from build123d import *

# Parameters (mm, degrees)
SKETCH1_W               = 1.5
SKETCH1_H               = 31
SKETCH1_W_2             = 2.5
SKETCH1_H_2             = 16
BOSS_EXTRUDE1_DEPTH     = 20
SKETCH2_W               = 70
SKETCH2_H               = 36
BOSS_EXTRUDE2_DEPTH     = 3
CUT_EXTRUDE1_DEPTH      = 82.215762017
CUT_EXTRUDE1_DEPTH_BACK = 82.215762017


with BuildPart() as part:
    # Sketch1 → Boss-Extrude1 (new body)
    with BuildSketch(Plane(origin=(0, 0, 0), x_dir=(1, 0, 0), z_dir=(0, 1, 0))):
        Polygon((70, 36), (0, 36), (0, 33.5), (68.5, 33.5), (70, 33.5), align=None)
        with Locations((69.25, 18)):
            Rectangle(SKETCH1_W, SKETCH1_H)
        Polygon((70, 0), (70, 2.5), (68.5, 2.5), (0, 2.5), (0, 0), align=None)
        with Locations((1.25, 18)):
            Rectangle(SKETCH1_W_2, SKETCH1_H_2)
    extrude(amount=BOSS_EXTRUDE1_DEPTH)

    # Sketch2 → Boss-Extrude2 (add)
    with BuildSketch(Plane.XZ):
        with Locations((35, -18)):
            Rectangle(SKETCH2_W, SKETCH2_H)
    extrude(amount=BOSS_EXTRUDE2_DEPTH)

    # Sketch3 → Cut-Extrude1 (cut, two sides: drawn at the far end of the back side and taken through both)
    with BuildSketch(Plane.XY.offset(-CUT_EXTRUDE1_DEPTH_BACK)):
        with BuildLine():
            Line((15, 3), (20, 3))
            ThreePointArc((20, 3), (21.5, 1.5), (20, 0))
            Line((20, 0), (15, 0))
            ThreePointArc((15, 0), (13.5, 1.5), (15, 3))
        make_face()
        with BuildLine():
            Line((55, 3), (50, 3))
            ThreePointArc((50, 3), (48.5, 1.5), (50, 0))
            Line((50, 0), (55, 0))
            ThreePointArc((55, 0), (56.5, 1.5), (55, 3))
        make_face()
    extrude(amount=CUT_EXTRUDE1_DEPTH + CUT_EXTRUDE1_DEPTH_BACK, mode=Mode.SUBTRACT)


solid = part.part
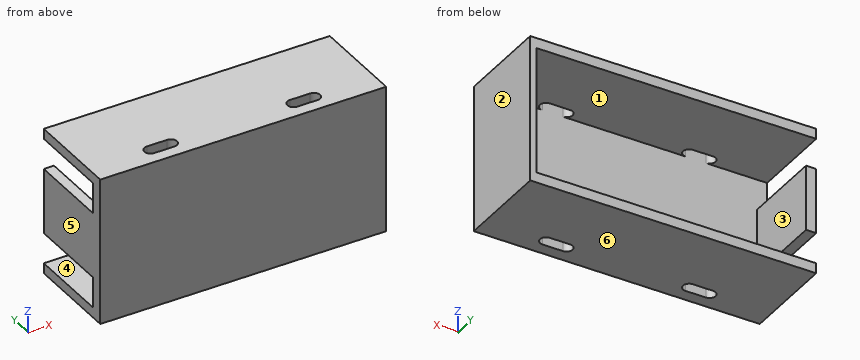
Here's how the part is built. I have some questions about the finished solid (model axes, mm). Face numbers are marked on the shaded views. A direction names the side the tool comes from. Coordinates: 2 decimals unless noted, no trailing zeros. Loops run counter-clockwise (first coordinate to the right, second up) from the corner with the lowest first, then second, coordinate; pieces in that order, holes last. Notation, with made-up numbers: (9, 87.5) -> (57, 87.5) arc R35 cw to (57, 121.5) -> close; hole circle Ø7 at (38, -27). An arc over 180 degrees is marked (long way). Use one line per item in the form item = value. Start each with the question number.
(1) If we section it at D-D (z = -4): Please give me the cut outline in (x, y).
(2) If we section it at C-C (x = 7): Please give me the cut outline in (y, z).
(3) We'd pull the mould along Z, two halves only. Please class the marked faces 4, 5 and 6: pulls with the +Z half, pulls with the -Z half, needs draft (parallel to the pull), parting line crosses it, or undercut.
(4) On a 3-axis mill with a long thin cutter (end or side, diameter ignored), from which of +Z, -Z, +X, -X, +Y, -Y can I reach the whole of each face in a straight line? I mean the marked faces 1, 2 and 3. Say none if no direction works.
(5) If we section it at A-A (y = 1.5): Please give me the cut outline in (x, z), then the cut area to 4 significant figures.
(6) If we section it at B-B (y = 18.25): Please give me the cut outline in (x, z), then the cut area to 4 significant figures.
(7) Please list where these lines run through material, in increasing order: line 1 along Z through (x, y) = (62, 14); line 2 along X through (y, z) = (1.5, -22.5); line 3 along Y through (x, z) = (49, -15).
(8) Will these pins go through, and if not, where does the flat tip stop? pin 1 (8 mm diameter, centred on x = 35.5, z = -13, fed in from +Y); pin 2 (3 mm diameter, centred on x = 1, y = 12.5, fed in from +Z); pin 3 (1 mm diameter, centred on y = 7, z = -27.5, fed in from -X).
Verdict:
q1.outline = (0, -3) -> (70, -3) -> (70, 20) -> (68.5, 20) -> (68.5, 0) -> (0, 0) -> close
q2.outline = (-3, -36) -> (20, -36) -> (20, -33.5) -> (0, -33.5) -> (0, -2.5) -> (20, -2.5) -> (20, 0) -> (-3, 0) -> close
q3.face_4 = undercut
q3.face_5 = needs draft
q3.face_6 = pulls with the -Z half
q4.face_1 = -X, +Y
q4.face_2 = +Z, -Z, +X, +Y, -Y
q4.face_3 = +Y
q5.outline = (0, -36) -> (13.5, -36) -> (13.5, -33.5) -> (0, -33.5) -> close; (0, -26) -> (2.5, -26) -> (2.5, -10) -> (0, -10) -> close; (0, -2.5) -> (13.5, -2.5) -> (13.5, 0) -> (0, 0) -> close; (21.5, -36) -> (48.5, -36) -> (48.5, -33.5) -> (21.5, -33.5) -> close; (21.5, -2.5) -> (48.5, -2.5) -> (48.5, 0) -> (21.5, 0) -> close; (56.5, -36) -> (70, -36) -> (70, 0) -> (56.5, 0) -> (56.5, -2.5) -> (68.5, -2.5) -> (68.5, -33.5) -> (56.5, -33.5) -> close
q5.area = 356.5 mm²
q6.outline = (0, -36) -> (70, -36) -> (70, 0) -> (0, 0) -> (0, -2.5) -> (68.5, -2.5) -> (68.5, -33.5) -> (0, -33.5) -> close; (0, -26) -> (2.5, -26) -> (2.5, -10) -> (0, -10) -> close
q6.area = 436.5 mm²
q7.line_1 = -36 to -33.5, -2.5 to 0
q7.line_2 = 0 to 2.5, 68.5 to 70
q7.line_3 = -3 to 0
q8.pin_1 = 0
q8.pin_2 = 0
q8.pin_3 = 68.5
